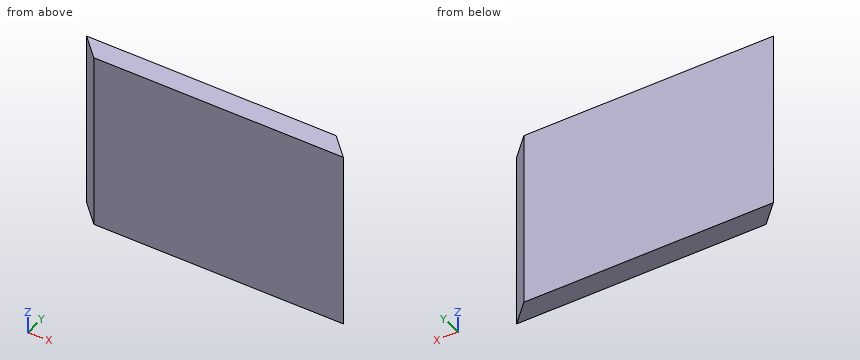
Autodesk Inventor part; units mm, degrees
ref_plane "YZ Plane" through (0, 0, 0) normal (1, 0, 0) x (0, 1, 0)
ref_plane "XZ Plane" through (0, 0, 0) normal (0, 1, 0) x (-1, 0, 0)
ref_plane "XY Plane" through (0, 0, 0) normal (0, 0, 1) x (1, 0, 0)
sketch "Sketch1" plane through (0, 0, 0) normal (0, 1, 0) x (-1, 0, 0)
  line L0 (-115, -80) -> (115, -80)
  line L1 (115, -80) -> (115, 80)
  line L2 (115, 80) -> (-115, 80)
  line L3 (-115, 80) -> (-115, -80)
  line L4 (-115, -80) -> (115, 80) construction
  line L5 (115, -80) -> (-115, 80) construction
  point P0 (0, 0)
  dimension "d0" = 230
  dimension "d1" = 160
extrude "Extrusion1" add sketch "Sketch1" along normal blind 20
chamfer "Chamfer1" distance 20 angle 45 1 edges at (115, 20, 0)
sketch "Sketch2" plane through (-115, 0, -80) normal (-1, 0, 0) x (0, 0, 1)
  line L0 (0, 20) -> (160, 20)
  line L1 (0, 20) -> (160, 20)
  line L2 (160, 20) -> (160, 0)
  line L3 (160, 0) -> (0, 0)
  line L4 (0, 0) -> (0, 20)
  point P0 (80, 0)
extrude "Extrusion2" add sketch "Sketch2" along normal blind 20
chamfer "Chamfer2" distance 20 angle 45 1 edges at (-135, 0, 0)
properties part number "FieldOfView" material "Titanium"
The model under review builds one solid part; all positions refer to its coordinate system, in mm. Round coordinates to 2 decimals unless told otherwise and drop trailing zeros. Order: outer loops, then holes, each group sorted by start corner. A loop starts at its lowest first (then second) coordinate and runs counter-clockwise, first axis right, second up. Notation, with made-up numbers: (22.25, -27.5) -> (70.25, -27.5) arc R19 cw to (70.25, -4.5) -> close; hole circle Ø7 at (48.25, 64). An arc over 180 degrees is marked (long way). Use a Markdown table: item, result.
Q1. For line 1 (X direction, y = 10.75, z = -50); line 2 (Y direction, x = 104, z = 15); line 3 (X direction, y = 18, z = 50), list the stretches that pass through material, from the lowest coordinate up.
Values:
| item | result |
|---|---|
| line 1 | x = -125.75 to 104.25 |
| line 2 | y = 0 to 11 |
| line 3 | x = -133 to 97 |
Q2. Clearance check with flat-ended pins moving along their axes: P1, Ø1, axis at y = 10.5, z = 9, coming from the +X side; P2, Ø4, axis at y = 3.5, z = 45, coming from the +X side; P3, Ø2, axis at y = 16, z = 44.5, coming from the +X side. State where each tip first meets the part, or that it passes through.
Values:
| item | result |
|---|---|
| P1 | stops at x = 105 |
| P2 | stops at x = 113.5 |
| P3 | stops at x = 100 |
Q3. We need section B-B on y = 12. Write out the cut boundary in (x, z).
Values:
| item | result |
|---|---|
| outline | (-127, -80) -> (103, -80) -> (103, 80) -> (-127, 80) -> close |
